The listing builds one solid part. Answer for the finished solid, in the listing's coordinates (mm). Coordinates: 2 decimals unless noted, no trailing zeros. Order: outer loops, then holes, each group sorted by start corner. A loop starts at its lowest first (then second) coordinate and runs counter-clockwise, first axis right, second up. Notation, with made-up numbers: (82.5, -4) - (140.5, -4) arc R17 ccw to (140.5, 26) - close; hole circle Ø1 at (23, -24.75). An arc over 180 degrees is marked (long way). One line per item, written item: value. Start each with the question number.
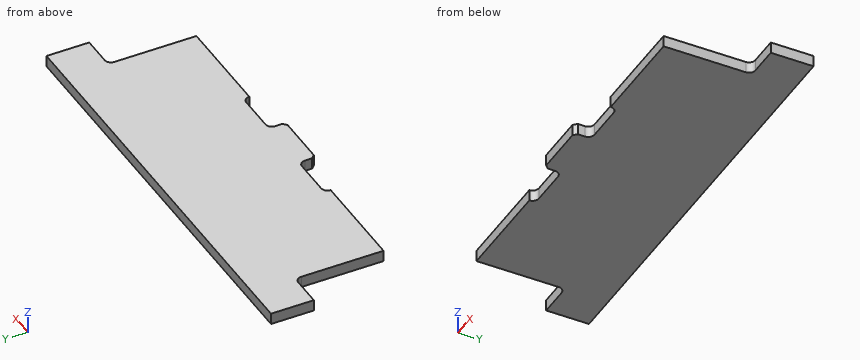
Autodesk Inventor part; units mm, degrees
ref_plane "YZ Plane" through (0, 0, 0) normal (1, 0, 0) x (0, 1, 0)
ref_plane "XZ Plane" through (0, 0, 0) normal (0, 1, 0) x (-1, 0, 0)
ref_plane "XY Plane" through (0, 0, 0) normal (0, 0, 1) x (1, 0, 0)
sketch "Sketch1" plane through (0, 0, 0) normal (0, 0, 1) x (1, 0, 0)
  line L0 (-30, 12.6375) -> (30, 12.6375)
  line L1 (30, 12.6375) -> (30, 6.6375)
  line L2 (30, 6.6375) -> (25.875, 6.6375)
  line L3 (25, 5.7625) -> (25, -5.7625)
  line L4 (25, -5.7625) -> (10.875, -5.7625)
  line L5 (4, -5.7625) -> (4, -6.7625)
  line L6 (3.5, -7.2625) -> (-3.5, -7.2625)
  line L7 (-4, -6.7625) -> (-4, -5.7625)
  line L8 (-10.875, -5.7625) -> (-25, -5.7625)
  line L9 (-25, -5.7625) -> (-25, 5.7625)
  line L10 (-25.875, 6.6375) -> (-30, 6.6375)
  line L11 (-30, 6.6375) -> (-30, 12.6375)
  arc A0 (-4, -5.7625) -> (-4.875, -4.8875) centre (-4.875, -5.7625) ccw
  arc A1 (4.875, -4.8875) -> (4, -5.7625) centre (4.875, -5.7625) ccw
  arc A2 (-25, 5.7625) -> (-25.875, 6.6375) centre (-25.875, 5.7625) ccw
  arc A3 (25.875, 6.6375) -> (25, 5.7625) centre (25.875, 5.7625) ccw
  line L12 (0, 4.2796) -> (0, -4.2796) construction
  line L13 (-9.9053, 0) -> (11.8635, 0) construction
  line L14 (-4, -6.7625) -> (-3.5, -7.2625)
  line L15 (3.5, -7.2625) -> (4, -6.7625)
  arc A4 (-10, -4.8875) -> (-10.875, -5.7625) centre (-10, -5.7625) ccw
  arc A5 (10.875, -5.7625) -> (10, -4.8875) centre (10, -5.7625) ccw
  line L16 (-10, -4.8875) -> (-4.875, -4.8875)
  line L17 (4.875, -4.8875) -> (10, -4.8875)
  point P0 (0, 0)
  point P1 (0, 12.6375)
  point P2 (-25, 0)
  dimension "d0" = 1.75
  dimension "d3" = 1.5
  dimension "d5" = 6
  dimension "d6" = 5
  dimension "d11" = 25
  dimension "d12" = 45
  dimension "d13" = 0.5
  dimension "d14" = 8
  dimension "d16" = 18.4
  dimension "d17" = 6
extrude "Extrusion1" add sketch "Sketch1" along normal blind 1.6
sketch "Sketch2" plane through (0, 0, 1.6) normal (0, 0, 1) x (1, 0, 0)
  line L0 (30, 12.6375) -> (-30, 12.6375)
  point P0 (0, 0)
  point P1 (-16, 2.1375)
  point P2 (0, 2.1375)
  point P3 (16, 2.1375)
  dimension "d9" = 16
  dimension "d10" = 16
  dimension "d15" = 10.5
properties part number "AK-C-C39-Insert-Board"
(1) Flat-ended cylindrical pins translate along their axes: pin 1 Ø0.5 at (x, z) = (-16, 1) entering from -Y; pin 2 Ø0.5 at (y, z) = (3, 1) entering from +X; pin 3 Ø0.8 at (x, z) = (-28.5, 1) entering from -Y. Find the tip coordinate at first contact, or state that the pin passes through.
(2) Consider probe 1 along X at (y, z) = (-0.5, 1.1); probe 2 along Y at (x, z) = (-8.5, 0.7); probe 3 along X at (y, z) = (-6, 0.55). Determine where each line is inside the solid, lowest interval first.
(3) The part is cut by section B-B on y = -1.5. Determine the outline of the cut face in (x, z).
(4) The part is cut by section C-C on x = -8. Determine the outline of the cut face in (y, z).
Completed:
1. pin 1: stops at y = -5.76
1. pin 2: stops at x = 25
1. pin 3: stops at y = 6.64
2. probe 1: x = -25 to 25
2. probe 2: y = -4.89 to 12.64
2. probe 3: x = -4 to 4
3. outline: (-25, 0) - (25, 0) - (25, 1.6) - (-25, 1.6) - close
4. outline: (-4.89, 0) - (12.64, 0) - (12.64, 1.6) - (-4.89, 1.6) - close
